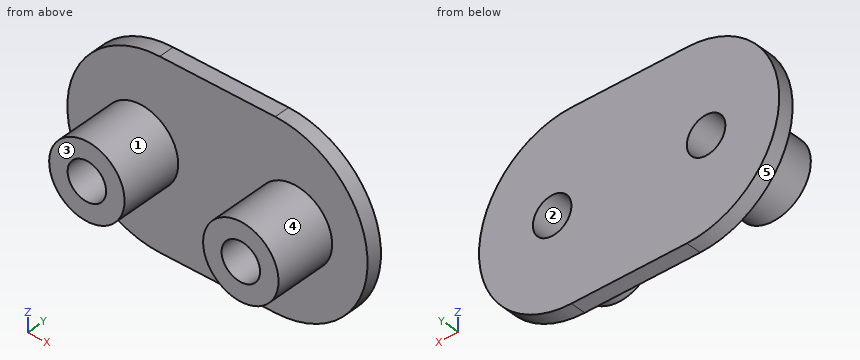
```python
from build123d import *

# Parameters (mm, degrees)
SKETCH1_R                  = 4.9
BOSS_EXTRUDE1_DEPTH        = 2
BOSS_EXTRUDE2_DEPTH        = 2
BOSS_EXTRUDE2_DEPTH_BACK   = 8
SKETCH1_3_R                = 4.9
SKETCH1_3_R_2              = 2.5
BOSS_EXTRUDE2_2_DEPTH      = 2
BOSS_EXTRUDE2_2_DEPTH_BACK = 8
SKETCH2_R                  = 5.756408641
SKETCH2_R_2                = 3.886057863
SKETCH2_R_3                = 6.078413945
SKETCH2_R_4                = 3.85710511
BOSS_EXTRUDE3_DEPTH        = 2


with BuildPart() as part:
    # Sketch1 → Boss-Extrude1 (new body)
    with BuildSketch(Plane(origin=(0, 0, 0), x_dir=(1, 0, 0), z_dir=(0, 1, 0))):
        with BuildLine():
            Line((-7.5, 12), (7.5, 12))
            ThreePointArc((7.5, 12), (19.5, 0), (7.5, -12))
            Line((7.5, -12), (-7.5, -12))
            ThreePointArc((-7.5, -12), (-19.5, 0), (-7.5, 12))
        make_face()
        with Locations(Location((-10, 0, 0), (0, 0, 270))):
            Circle(SKETCH1_R, mode=Mode.SUBTRACT)
        with Locations(Location((10, 0, 0), (0, 0, 270))):
            Circle(SKETCH1_R, mode=Mode.SUBTRACT)
    extrude(amount=BOSS_EXTRUDE1_DEPTH)



with BuildPart() as body_2:
    # Sketch1_3 → Boss-Extrude2 (new, two sides: drawn at the far end of the back side and taken through both)
    with BuildSketch(Plane(origin=(0, 0, 0), x_dir=(1, 0, 0), z_dir=(0, 1, 0)).offset(-BOSS_EXTRUDE2_DEPTH_BACK)):
        with Locations(Location((-10, 0, 0), (0, 0, 270))):
            Circle(SKETCH1_3_R)
        with Locations(Location((-10, 0, 0), (0, 0, 270))):
            Circle(SKETCH1_3_R_2, mode=Mode.SUBTRACT)
    extrude(amount=BOSS_EXTRUDE2_DEPTH + BOSS_EXTRUDE2_DEPTH_BACK)


with BuildPart() as body_3:
    # Sketch1_3 → Boss-Extrude2 2 (new, two sides: drawn at the far end of the back side and taken through both)
    with BuildSketch(Plane(origin=(0, 0, 0), x_dir=(1, 0, 0), z_dir=(0, 1, 0)).offset(-BOSS_EXTRUDE2_2_DEPTH_BACK)):
        with Locations(Location((10, 0, 0), (0, 0, 270))):
            Circle(SKETCH1_3_R)
        with Locations(Location((10, 0, 0), (0, 0, 270))):
            Circle(SKETCH1_3_R_2, mode=Mode.SUBTRACT)
    extrude(amount=BOSS_EXTRUDE2_2_DEPTH + BOSS_EXTRUDE2_2_DEPTH_BACK)


with BuildPart() as part_1:
    add(part.part)

    add(body_2.part)  # Boss-Extrude3 merges body 2

    add(body_3.part)  # Boss-Extrude3 merges body 3
    # Sketch2 → Boss-Extrude3 (add)
    # profile 1 of 2: a face of its own
    with BuildSketch(Plane(origin=(0, 2, 0), x_dir=(1, 0, 0), z_dir=(0, 1, 0))):
        with Locations((-10, 0)):
            Circle(SKETCH2_R)
        with Locations((-10, 0)):
            Circle(SKETCH2_R_2, mode=Mode.SUBTRACT)
    # profile 2 of 2: a face of its own
    with BuildSketch(Plane(origin=(0, 2, 0), x_dir=(1, 0, 0), z_dir=(0, 1, 0))):
        with Locations((10, 0)):
            Circle(SKETCH2_R_3)
        with Locations((10, 0)):
            Circle(SKETCH2_R_4, mode=Mode.SUBTRACT)
    extrude(amount=-BOSS_EXTRUDE3_DEPTH)


solid = part_1.part
```
Part model, mm, in its own coordinate system. Face numbers are marked on the shaded views. A direction names the side the tool comes from. Round coordinates to 2 decimals unless told otherwise and drop trailing zeros. Loops run counter-clockwise (first coordinate to the right, second up) from the corner with the lowest first, then second, coordinate; pieces in that order, holes last.
1. Slice it at A-A (z = 0). Give the cut face in (x, y).
Solutions:
outline: (-19.5, 0) - (-14.9, 0) - (-14.9, -8) - (-12.5, -8) - (-12.5, 2) - (-19.5, 2) - close; (-7.5, -8) - (-5.1, -8) - (-5.1, 0) - (5.1, 0) - (5.1, -8) - (7.5, -8) - (7.5, 2) - (-7.5, 2) - close; (12.5, -8) - (14.9, -8) - (14.9, 0) - (19.5, 0) - (19.5, 2) - (12.5, 2) - close
2. Flat gauge pins, fed straight in: pin 1 (5 mm diameter, centred on x = -15, y = -0.5, fed in from -Z); pin 2 (4.5 mm diameter, centred on x = -10, z = 0, fed in from +Y); pin 3 (3 mm diameter, centred on y = -5.5, z = -5.5, fed in from -X); pin 4 (1.5 mm diameter, centred on x = 10, z = -7.5, fed in from -Y). Where does each tip first touch, or does it go through?
Solutions:
pin 1: stops at z = -10.89
pin 2: passes through
pin 3: stops at x = -12.83
pin 4: stops at y = 0
3. 3-axis set-ups, long thin cutter, end or side, ignore diameter. For the marked faces 1 and 2: which of +Z, -Z, +X, -X, +Y, -Y reach the whole face in a straight line?
Solutions:
face 1: -Y
face 2: +Y, -Y
4. Slice it at D-D (y = -5). Give the cut face in (x, z), and give its area (3 significant figures).
Solutions:
outline: circle Ø9.8 at (-10, 0); circle Ø9.8 at (10, 0); hole circle Ø5 at (-10, 0); hole circle Ø5 at (10, 0)
area: 112 mm2
5. Slice it at C-C (x = 10.5). Give the cut face in (y, z), and give its area (3 significant figures).
Solutions:
outline: (-8, -4.87) - (0, -4.87) - (0, -11.62) - (2, -11.62) - (2, -2.45) - (-8, -2.45) - close; (-8, 2.45) - (2, 2.45) - (2, 11.62) - (0, 11.62) - (0, 4.87) - (-8, 4.87) - close
area: 75.5 mm2
6. Two-plate mould, pull along X, no slides. Class the marked faces 3, 4 and 5: pulls with the +X half, pulls with the -X half, needs draft (parallel to the pull), parting line crosses it, or undercut.
Solutions:
face 3: needs draft
face 4: undercut
face 5: pulls with the -X half
7. Slice it at B-B (y = 0.5). Give the cut face in (x, z).
Solutions:
outline: (-7.5, -12) - (7.5, -12) arc R12 ccw to (7.5, 12) - (-7.5, 12) arc R12 ccw to start; hole circle Ø5 at (-10, 0); hole circle Ø5 at (10, 0)
8. Drill centre lines: line 1 along X through (y, z) = (-2.25, 0); line 2 along X through (y, z) = (-5.5, 3); line 3 along Y through (x, z) = (15.5, 1.5). Where is each one in solid material? Low to high.
Solutions:
line 1: x = -14.9 to -12.5, -7.5 to -5.1, 5.1 to 7.5, 12.5 to 14.9
line 2: x = -13.87 to -6.13, 6.13 to 13.87
line 3: y = 0 to 2
